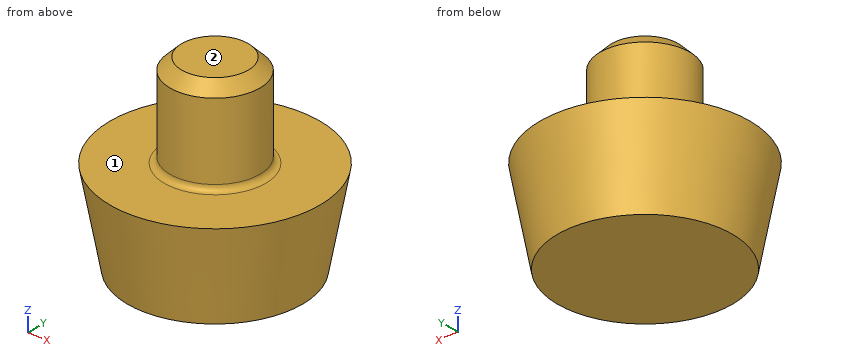
Autodesk Fusion 360 part; units mm, degrees
sketch "Sketch1" plane through (0, 0, 0) normal (0, 1, 0) x (1, 0, 0)
  line L0 (0, 0) -> (7.5, 0)
  line L1 (7.5, 0) -> (9, -8)
  line L2 (9, -8) -> (4.35, -8)
  line L3 (3.85, -8.5) -> (3.85, -16)
  line L4 (3.85, -16) -> (0, -16)
  line L5 (0, -16) -> (0, 0)
  arc A0 (4.35, -8) -> (3.85, -8.5) centre (4.35, -8.5) ccw
  point P0 (3.85, -8)
  dimension "d1" = 7.5
  dimension "d2" = 8
  dimension "d3" = 3.85
  dimension "d4" = 8
  dimension "d5" = 0.5
revolve "Revolve1" add sketch "Sketch1" angle 360 about axis through (0, 0, 16) along (0, 0, -1)
chamfer "Chamfer1" distance 1 angle 45 1 edges at (-3.5895, -1.3922, 16)
Read the model definition and answer for the solid it produces. Units are mm, in the model's axes. Face numbers are marked on the shaded views. A direction names the side the tool comes from. Give positions to 0.01 mm unless a question says otherwise; leave off trailing zeros. Loops run counter-clockwise (first coordinate to the right, second up) from the corner with the lowest first, then second, coordinate; pieces in that order, holes last. Notation, with made-up numbers: (27.5, 87.5) - (44.5, 87.5) arc R4 ccw to (44.5, 93.5) - close; hole circle Ø7 at (19, -15.5). An arc over 180 degrees is marked (long way). Answer as CSV lines item,"result". Start each with the question number.
1) Find section C-C (z = 14). Write down the section's boundary in (x, y), then the cut area to 3 significant figures.
2) Find section A-A (y = 0). Write down the section's boundary in (x, z), then the cut area to 3 significant figures.
3) Straight lines are drawn through the part: L1, parallel to Z at x = 5.75, y = 3.75; L2, parallel to Y at x = 0, z = 9.25; L3, parallel to Y at x = 1, z = 4.25. For each, find the intervals that lie inside material, in ascending order. Write a range as from..to.
4) Find section D-D (z = 5.25). Write down the section's boundary in (x, y).
5) Which of the six approach directions +Z, -Z, +X, -X, +Y, -Y give full straight-line access (tool end or side, diameter ignored) to the marked faces 1 and 2?
6) Each of these flat-tipped pins is pushed along its axis until it touches: pin 1 Ø8 at (y, z) = (-6.5, 4.5) entering from +X; pin 2 Ø4 at (x, z) = (-1, 4.5) entering from +Y; pin 3 Ø5 at (y, z) = (-6.5, 6) entering from -X. Where does it stop, or does it pass through?
Findings below:
1,outline,"circle Ø7.7 at (0, 0)"
1,area,"46.6 mm^2"
2,outline,"(-9, 8) - (-7.5, 0) - (7.5, 0) - (9, 8) - (4.35, 8) arc R0.5 cw to (3.85, 8.5) - (3.85, 15) - (2.85, 16) - (-2.85, 16) - (-3.85, 15) - (-3.85, 8.5) arc R0.5 cw to (-4.35, 8) - close"
2,area,"193 mm^2"
3,L1,"0..8"
3,L2,"-3.85..3.85"
3,L3,"-8.24..8.24"
4,outline,"circle Ø16.97 at (0, 0)"
5,face 1,"+Z"
5,face 2,"+Z, +X, -X, +Y, -Y"
6,pin 1,"x = 8.17"
6,pin 2,"y = 8.69"
6,pin 3,"x = -7.74"
